The drawing under review shows one solid part. Ordinate dimensions are in mm from its lowest x, y, z. A direction names the side the tool comes from. Round coordinates to 2 decimals unless told otherwise and drop trailing zeros. Order: outer loops, then holes, each group sorted by start corner. A loop starts at its lowest first (then second) coordinate and runs counter-clockwise, first axis right, second up. Notation, with made-up numbers: M 80,40.5 L 115,40.5 A14 cw 115,58.5 Z; hole C -35,42 d5. An arc over 180 degrees is marked long. Answer as a JSON object with one key per item and string values. Group by question number.
1. Mouldability with a two-part tool opening along X and no side actions: class the marked faces 4, 5, 6 and 7 as released by +X, released by -X, zero draft, split by the parting line, or undercut.
2. Machinability: for the marked faces 1, 2 and 3, which of the approach directions +Z, -Z, +X, -X, +Y, -Y give a long, thin tool a straight path to every point of the face, cutting with its end or side? Answer none if there is none.
3. Add section C-C on x = 27.5. State the section outline as (y, z) points, and give its area (3 significant figures).
4. Add section B-B on y = 15. State the section outline as (x, z) points.
5. To check wall thickness, follow probe 1 along X at (y, z) = (25, 1.5); probe 2 along X at (y, z) = (6, 1.5); probe 3 along X at (y, z) = (15, 0.5). State the ranges of each line that lie inside material, in increasing order. Write a range as [from, to].
6. Add section A-A on z = 6.5. State the section outline as (x, y) points, and give its area (3 significant figures).
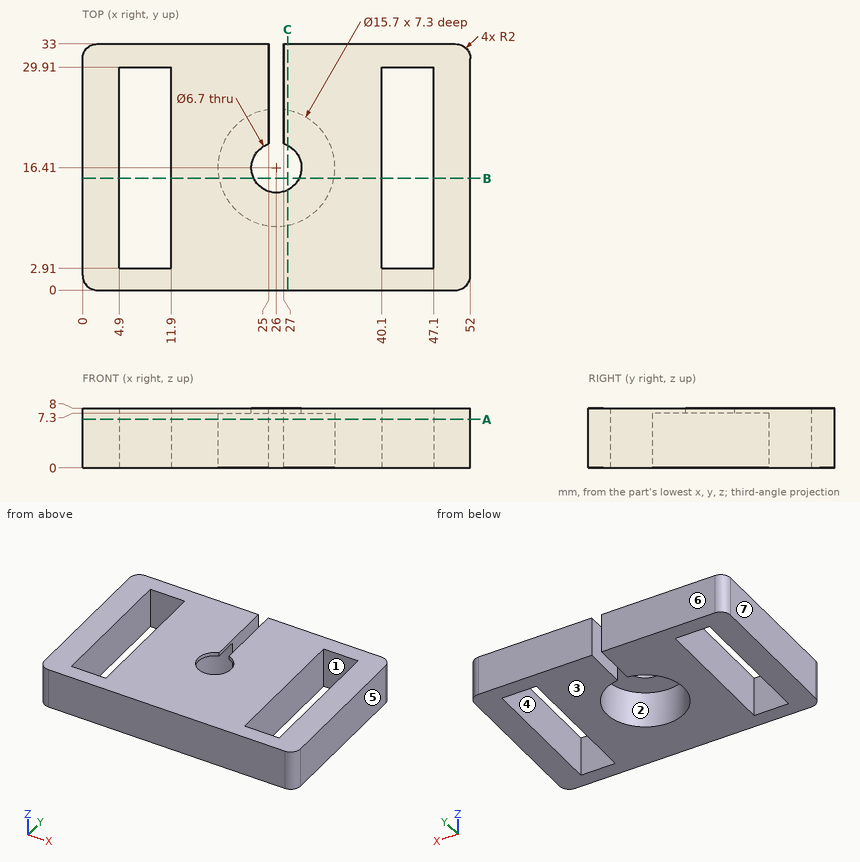
Recorded:
{
 "1": {"face 4": "undercut", "face 5": "released by +X", "face 6": "zero draft", "face 7": "released by -X"},
 "2": {"face 1": "+Z, -Z", "face 2": "-Z", "face 3": "-Z, +X, -X, +Y, -Y"},
 "3": {"outline": "M 0,0 L 8.7,0 L 8.7,7.3 L 13.41,7.3 L 13.41,8 L 0,8 Z; M 19.41,7.3 L 24.12,7.3 L 24.12,0 L 33,0 L 33,8 L 19.41,8 Z", "area": "147 mm²"},
 "4": {"outline": "M 0,0 L 4.9,0 L 4.9,8 L 0,8 Z; M 11.9,0 L 18.28,0 L 18.28,7.3 L 22.96,7.3 L 22.96,8 L 11.9,8 Z; M 29.04,7.3 L 33.72,7.3 L 33.72,0 L 40.1,0 L 40.1,8 L 29.04,8 Z; M 47.1,0 L 52,0 L 52,8 L 47.1,8 Z"},
 "5": {"probe 1": "x = [0, 4.9], [11.9, 25], [27, 40.1], [47.1, 52]", "probe 2": "x = [0, 4.9], [11.9, 40.1], [47.1, 52]", "probe 3": "x = [0, 4.9], [11.9, 18.28], [33.72, 40.1], [47.1, 52]"},
 "6": {"outline": "M 0,2 A2 ccw 2,0 L 50,0 A2 ccw 52,2 L 52,31 A2 ccw 50,33 L 27,33 L 27,24.2 A7.85 cw long 25,24.2 L 25,33 L 2,33 A2 ccw 0,31 Z; hole M 4.9,2.91 L 11.9,2.91 L 11.9,29.91 L 4.9,29.91 Z; hole M 40.1,2.91 L 47.1,2.91 L 47.1,29.91 L 40.1,29.91 Z", "area": "1,120 mm²"}
}
